```python
from build123d import *

# Parameters (mm, degrees)
F1_DEPTH      = 3
F3_DEPTH      = 70
F3_DEPTH_BACK = 70
F4_DEPTH      = 1.5
F6_DEPTH      = 1.5


with BuildPart() as f1:
    # F0 (on Front) → F1 (new body)
    with BuildSketch(Plane.XZ):
        Polygon((-54.177348, 139.05524), (-65, 113.442006), (-2, 113.442006), (-2, 125.442006), (2, 125.442006), (2, 113.442006), (65, 113.442006), (56.497385, 133.564567), (41.497385, 133.564567), (0, 267.273082), align=None)
        Polygon((-67.99451, 144.893563), (-54.177348, 139.05524), (0, 267.273082), align=None)
        Polygon((56.497385, 133.564567), (0, 267.273082), (41.497385, 133.564567), align=None)
    extrude(amount=F1_DEPTH)

    # F2 (on face) → F3 (cut, two sides)
    with BuildSketch(Plane.YZ.offset(-2)) as f3_sk:
        with BuildLine():
            ThreePointArc((-1.5, 114.442006), (-1.146447, 114.588452), (-1, 114.942006))
            ThreePointArc((-1, 114.942006), (-1.5, 115.442006), (-2, 114.942006))
            ThreePointArc((-2, 114.942006), (-1.853553, 114.588452), (-1.5, 114.442006))
        make_face()
    extrude(amount=F3_DEPTH, mode=Mode.SUBTRACT)
    extrude(f3_sk.sketch, amount=-F3_DEPTH_BACK, mode=Mode.SUBTRACT)

    # F0 (on Front) → F4 (cut)
    with BuildSketch(Plane.XZ):
        Polygon((56.497385, 133.564567), (0, 267.273082), (41.497385, 133.564567), align=None)
    extrude(amount=F4_DEPTH, mode=Mode.SUBTRACT)

    # F5 (on face) → F6 (cut)
    with BuildSketch(Plane.XZ.offset(3)):
        Polygon((-67.99451, 144.893563), (-54.177348, 139.05524), (0, 267.273082), align=None)
    extrude(amount=-F6_DEPTH, mode=Mode.SUBTRACT)


solid = f1.part
```
Verification items for the finished model (mm, model axes). A direction names the side the tool comes from. Coordinates: 2 decimals unless noted, no trailing zeros. Order: outer loops, then holes, each group sorted by start corner. A loop starts at its lowest first (then second) coordinate and runs counter-clockwise, first axis right, second up. Notation, with made-up numbers: (70.25, 17.5) -> (126.25, 17.5) arc R13 ccw to (126.25, 31.5) -> close; hole circle Ø7 at (3.25, 38.5). An arc over 180 degrees is marked (long way). Answer as CSV lines item,"result". Start each with the question number.
1) Cross-section at A-A, the plane x = 37.5. Record the boundary of the cut face in (y, z), then the cut area to 3 significant figures.
2) Cross-section at C-C, the plane x = 5. Record the boundary of the cut face in (y, z), then the cut area to 3 significant figures.
3) Cross-section at B-B, the plane z = 257. Record the boundary of the cut face in (x, y).
4) Gauge pin test, flat ends, axial feed: pin 1 Ø1 at (y, z) = (-1.5, 238.5) entering from -X; pin 2 Ø1.6 at (x, y) = (47.5, -0.5) entering from +Z; pin 3 Ø0.9 at (y, z) = (-1.5, 119) entering from -X. Record the tip position at first contact, or that the pin passes through.
5) Release check for a two-part mould opening along Z. For faces 4 (the face through (-2, 0, 174)), 5 (the face through (-33.52, -0.74, 206.94)), 6 (the face through (-61.183, -0.74, 142.015)) record: released by +Z, released by -Z, zero draft, split by the parting line, or undercut.
6) Set-up check for faces 1 (the face through (32, -1.5, 176)), 2 (the face through (-1, -3, 174)), 3 (the face through (-39, -1.5, 184)): record each of +Z, -Z, +X, -X, +Y, -Y from which the full face is reachable in a straight line by a thin tool's end or side.
7) Cross-section at D-D, the plane z = 163. Record the boundary of the cut face in (x, y), then the cut area to 3 significant figures.
8) Material ranges on L1, parallel to Z at x = -60, y = -1.25; L2, parallel to Z at x = 50, y = -1.4; L3, parallel to X at y = -1.4, z = 120.5, recorded low to high. Write a range as [from, to].
Conclusion:
1,outline,"(-3, 113.44) -> (0, 113.44) -> (0, 146.44) -> (-1.5, 146.44) -> (-1.5, 178.52) -> (-3, 178.52) -> close; hole circle Ø1 at (-1.5, 114.94)"
1,area,"146 mm²"
2,outline,"(-3, 113.44) -> (0, 113.44) -> (0, 251.16) -> (-1.5, 251.16) -> (-1.5, 255.44) -> (-3, 255.44) -> close; hole circle Ø1 at (-1.5, 114.94)"
2,area,"419 mm²"
3,outline,"(-5.71, -1.5) -> (-4.34, -1.5) -> (-4.34, -3) -> (4.34, -3) -> (4.34, -1.5) -> (3.19, -1.5) -> (3.19, 0) -> (-5.71, 0) -> close"
4,pin 1,"stops at x = -16.26"
4,pin 2,"stops at z = 133.56"
4,pin 3,"stops at x = -62.84"
5,face 4,"zero draft"
5,face 5,"released by +Z"
5,face 6,"undercut"
6,face 1,"+Z, +X, +Y"
6,face 2,"+Z, -Z, +X, -X, -Y"
6,face 3,"+Z, -X, -Y"
7,outline,"(-57.93, -1.5) -> (-44.06, -1.5) -> (-44.06, -3) -> (44.06, -3) -> (44.06, -1.5) -> (32.36, -1.5) -> (32.36, 0) -> (-57.93, 0) -> close"
7,area,"268 mm²"
8,L1,"z = [113.44, 114.51], [115.38, 125.28], [141.52, 159.28]"
8,L2,"z = [113.44, 114.45], [115.43, 133.56]"
8,L3,"x = [-62.02, -2], [2, 62.02]"
